from build123d import *

# Parameters (mm, degrees)
BOSS_EXTRUDE1_DEPTH = 6
CUT_EXTRUDE1_DEPTH  = 91.068866014
SKETCH4_R           = 2.5
HOLE1_DEPTH         = 91.068866014
SKETCH5_R           = 2.5
HOLE2_DEPTH         = 91.068866014


with BuildPart() as part:
    # Sketch2 → Boss-Extrude1 (new body)
    with BuildSketch(Plane.XY):
        with BuildLine():
            Line((-56.975, 0), (56.975, 0))
            Line((56.975, 0), (56.975, 57.1))
            ThreePointArc((56.975, 57.1), (53.343124087, 65.868124087), (44.575, 69.5))
            Line((44.575, 69.5), (-44.575, 69.5))
            ThreePointArc((-44.575, 69.5), (-53.343124087, 65.868124087), (-56.975, 57.1))
            Line((-56.975, 57.1), (-56.975, 0))
        make_face()
    extrude(amount=BOSS_EXTRUDE1_DEPTH)

    # Sketch3 → Cut-Extrude1 (cut, through all)
    with BuildSketch(Plane.XY.offset(6)):
        Polygon((-40.55, 0), (-35.55, 0), (-35.55, 6.05), (-33.175, 6.05), (-33.175, 10.8), (-35.55, 10.8), (-35.55, 14.6), (-40.55, 14.6), (-40.55, 10.8), (-42.925, 10.8), (-42.925, 6.05), (-40.55, 6.05), align=None)
    cut_extrude1 = extrude(amount=-CUT_EXTRUDE1_DEPTH, mode=Mode.SUBTRACT)

    # Sketch4 → Hole1 (cut, through all)
    with BuildSketch(Plane.XY.offset(6)):
        with Locations((-45.825, 41)):
            Circle(SKETCH4_R)
    hole1 = extrude(amount=-HOLE1_DEPTH, mode=Mode.SUBTRACT)

    # Sketch5 → Hole2 (cut, through all)
    with BuildSketch(Plane.XY.offset(6)):
        with Locations((0, 58.3)):
            Circle(SKETCH5_R)
    extrude(amount=-HOLE2_DEPTH, mode=Mode.SUBTRACT)

    # Mirror1: Cut-Extrude1, Hole1 across plane
    add(cut_extrude1.mirror(Plane(origin=(0, 0, 0), x_dir=(0, 0, 1), z_dir=(1, 0, 0))), mode=Mode.SUBTRACT)
    add(hole1.mirror(Plane(origin=(0, 0, 0), x_dir=(0, 0, 1), z_dir=(1, 0, 0))), mode=Mode.SUBTRACT)


solid = part.part
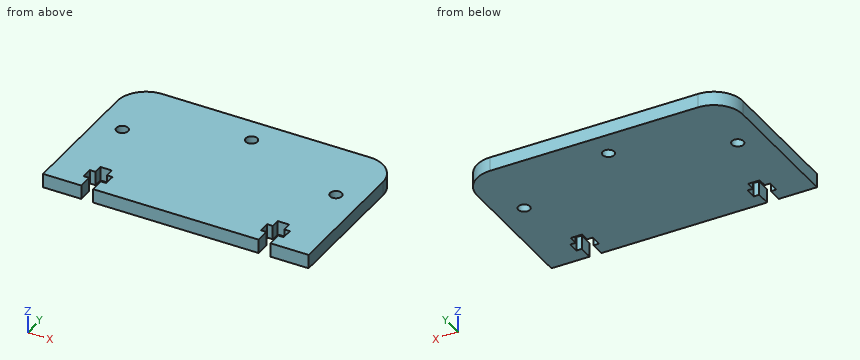
Geometry check sheet. Reference: the model listing, model coordinates, mm. Round coordinates to 2 decimals unless told otherwise and drop trailing zeros. Loops run counter-clockwise (first coordinate to the right, second up) from the corner with the lowest first, then second, coordinate; pieces in that order, holes last. Notation, with made-up numbers: (-37, -20) - (21, -20) arc R27 ccw to (21, -4) - close; hole circle Ø4 at (68.25, 34). An arc over 180 degrees is marked (long way). Answer as CSV lines item,"result".
(1) Cross-section at D-D, the plane y = 58.3. Enter the section's corners in (x, z).
Output values:
outline,"(-56.92, 0) - (-2.5, 0) - (-2.5, 6) - (-56.92, 6) - close; (2.5, 0) - (56.92, 0) - (56.92, 6) - (2.5, 6) - close"
(2) Depth check by flat-ended pin: pin 1 Ø6 at (x, y) = (0, 58.3) entering from +Z; pin 2 Ø3 at (y, z) = (61, 1) entering from +X; pin 3 Ø2.5 at (x, z) = (38.5, 3.5) entering from -Y; pin 4 Ø2 at (y, z) = (61.5, 1.5) entering from +X. Enter the tip coordinate at first touch or a pass-through.
Output values:
pin 1,"stops at z = 6"
pin 2,"stops at x = 56.74"
pin 3,"stops at y = 14.6"
pin 4,"stops at x = 56.5"
(3) Cross-section at B-B, the plane y = 41. Enter the section's corners in (x, z) (3 decimals).
Output values:
outline,"(-56.975, 0) - (-48.325, 0) - (-48.325, 6) - (-56.975, 6) - close; (-43.325, 0) - (43.325, 0) - (43.325, 6) - (-43.325, 6) - close; (48.325, 0) - (56.975, 0) - (56.975, 6) - (48.325, 6) - close"
(4) Material ranges on line 1 along X through (y, z) = (9.5, 0.65) (3 decimals); line 2 along X through (y, z) = (39, 1.6) (3 decimals); line 3 along Y through (x, z) = (37, 5.55), recorded low to high.
Output values:
line 1,"x = -56.975 to -42.925, -33.175 to 33.175, 42.925 to 56.975"
line 2,"x = -56.975 to -47.325, -44.325 to 44.325, 47.325 to 56.975"
line 3,"y = 14.6 to 69.5"
(5) Cross-section at C-C, the plane z = 2.8. Give the number of separate pieces and of enclosed holes in the cut face, and give its area (3 significant figures).
Output values:
separate pieces,"1"
enclosed holes,"3"
area,"7,600 mm²"
(6) Cross-section at A-A, the plane x = 0. Enter the section's corners in (y, z), and give its area (3 significant figures).
Output values:
outline,"(0, 0) - (55.8, 0) - (55.8, 6) - (0, 6) - close; (60.8, 0) - (69.5, 0) - (69.5, 6) - (60.8, 6) - close"
area,"387 mm²"
